from build123d import *

# Parameters (mm, degrees)
SKETCH2_R          = 1
CUT_EXTRUDE1_DEPTH = 21.420577857
CIRPATTERN2_COUNT  = 8
SKETCH3_R          = 1
CUT_EXTRUDE2_DEPTH = 21.420577857
CIRPATTERN3_COUNT  = 4
CHAMFER1_SIZE      = 0.3


with BuildPart() as part:
    # Sketch1 → Revolve1 (revolve)
    with BuildSketch(Plane.XY, mode=Mode.PRIVATE) as revolve1_sk:
        Polygon((-5, 3.75), (-2, 3.75), (-2, 14), (0, 14), (0, 3), (-4.5, 3), (-4.5, 1.5), (-5, 1.5), align=None)
    revolve(revolve1_sk.sketch.rotate(Axis((0, 0, 0), (1, 0, 0)), 90), axis=Axis((0, 0, 0), (1, 0, 0)))

    # Sketch2 → Cut-Extrude1 (cut, through all)
    with BuildSketch(Plane(origin=(0, 0, 0), x_dir=(0, 0, -1), z_dir=(1, 0, 0))):
        with Locations((0, 11)):
            Circle(SKETCH2_R)
    cut_extrude1 = extrude(amount=-CUT_EXTRUDE1_DEPTH, mode=Mode.SUBTRACT)

    # CirPattern2: Cut-Extrude1 ×8 about axis
    cirpattern2_axis = Axis((0, 0, 0), (1, 0, 0))
    for i in range(1, CIRPATTERN2_COUNT):
        add(cut_extrude1.rotate(cirpattern2_axis, i * 360 / CIRPATTERN2_COUNT), mode=Mode.SUBTRACT)

    # Sketch3 → Cut-Extrude2 (cut, through all)
    with BuildSketch(Plane(origin=(0, 0, 0), x_dir=(0, 0, -1), z_dir=(1, 0, 0))):
        with Locations((0, 8)):
            Circle(SKETCH3_R)
    cut_extrude2 = extrude(amount=-CUT_EXTRUDE2_DEPTH, mode=Mode.SUBTRACT)

    # CirPattern3: Cut-Extrude2 ×4 about axis
    cirpattern3_axis = Axis((0, 0, 0), (1, 0, 0))
    for i in range(1, CIRPATTERN3_COUNT):
        add(cut_extrude2.rotate(cirpattern3_axis, i * 360 / CIRPATTERN3_COUNT), mode=Mode.SUBTRACT)

    # Chamfer1
    chamfer1_edges = [part.edges().sort_by_distance(p)[0] for p in [
        (-2, 11, 1),
        (-2, 8.485281374, -7.071067812),
        (-2, 1, -11),
        (-2, -7.071067812, -8.485281374),
        (-2, -11, -1),
        (-2, -8.485281374, 7.071067812),
        (-2, -1, 11),
        (-2, 7.071067812, 8.485281374),
        (-2, 8, 1),
        (-2, 1, -8),
        (-2, -8, -1),
        (-2, -1, 8),
        (-2, 0, -14),
        (-2, 0, -3.75),
        (-5, 0, -3.75),
    ]]
    chamfer(chamfer1_edges, length=CHAMFER1_SIZE)


solid = part.part
Work out the finished part from the listing and answer in its coordinate system (mm). A direction names the side the tool comes from. Coordinates: 2 decimals unless noted, no trailing zeros. Write each loop counter-clockwise with the first axis right and the second up, starting at its lowest first coordinate (ties: lowest second). Pieces come first, ordered by that corner, then holes.
1. For faces 4 (the cylindrical face through (-1, 9, 0)), 5 (the cylindrical face through (-2.28, -0.9, 2.86)), determine the directions among +Z, -Z, +X, -X, +Y, -Y from which every point of the face is accessible in a straight line to the end or side of a thin tool.
Results list:
face 4: +X, -X
face 5: +X
2. For a pull along Z with two mould halves and no side action, classify faces 1 (the cylindrical face through (-0.8, 12.4, 6.5)), 2 (the flat face through (-2, -3, 3)), 3 (the cylindrical face through (-0.838, -7.909, 6.787)) as +Z half, -Z half, draft (parallel to the pull), parting line (faces both ways), or undercut.
Results list:
face 1: parting line
face 2: draft
face 3: undercut
3. The part is cut by section C-C, the plane x = -3.9. Write down the section's boundary in (y, z), and give its area (3 significant figures).
Results list:
outline: circle Ø7.5 at (0, 0); hole circle Ø6 at (0, 0)
area: 15.9 mm2
4. Consider line 1 along X through (y, z) = (-2.75, -9.25); line 2 along Y through (x, z) = (-2.6, 2); line 3 along Y through (x, z) = (-1.05, -11). Determine where each line is inside the solid, lowest interval first.
Results list:
line 1: x = -2 to 0
line 2: y = -3.17 to -2.24, 2.24 to 3.17
line 3: y = -8.66 to -1, 1 to 8.66
5. Flat-ended cylindrical pins translate along their axes: pin 1 (2.5 mm diameter, centred on y = -7.78, z = -7.78, fed in from -X); pin 2 (1.8 mm diameter, centred on y = -1, z = -1.5, fed in from +X); pin 3 (1.5 mm diameter, centred on x = -2.5, y = -9.5, fed in from -Z). Find the tip coordinate at first contact, or state that the pin passes through.
Results list:
pin 1: stops at x = -1.95
pin 2: stops at x = -4.5
pin 3: stops at z = -10.42
6. The part is cut by section A-A, the plane x = -1.25. State how many separate pieces and enclosed holes the cut face has, and give its area (3 significant figures).
Results list:
separate pieces: 1
enclosed holes: 13
area: 550 mm2
